For this review, use the dimensioned drawing (mm, ordinates from the lowest corner) and the shaded views. Coordinates: 2 decimals unless noted, no trailing zeros. Loops run counter-clockwise (first coordinate to the right, second up) from the corner with the lowest first, then second, coordinate; pieces in that order, holes last. Notation, with made-up numbers: (17.5, 15) -> (30.5, 15) arc R30 ccw to (30.5, 40) -> close; hole circle Ø1 at (53, 44.5). An arc over 180 degrees is marked (long way). Answer as a JSON object with one key per item and string values.
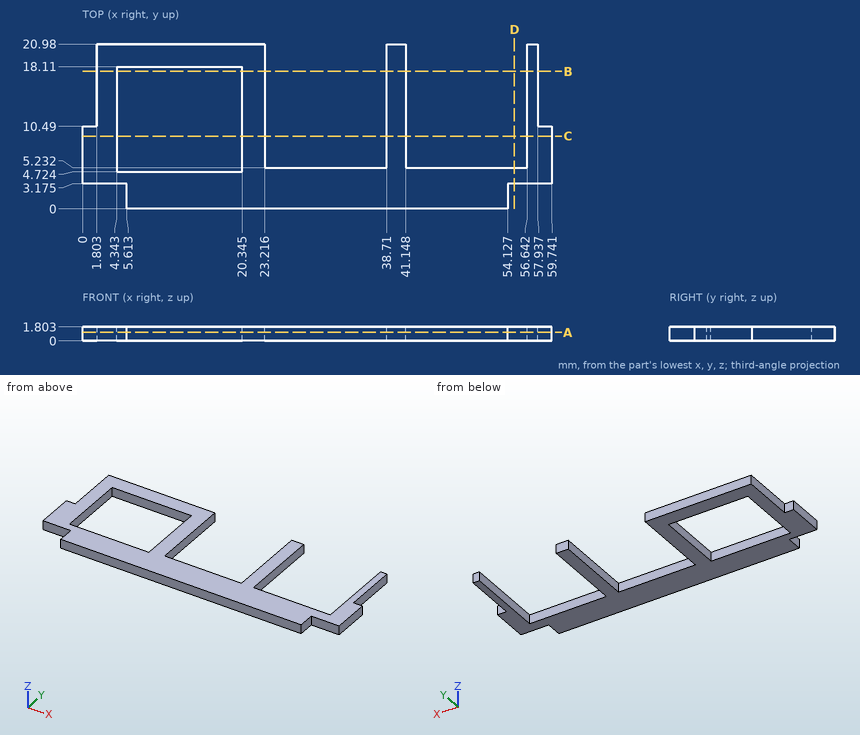
1) Wall thickness on probe 1 along X at (y, z) = (7.5, 1.15) (1 decimal); probe 2 along X at (y, z) = (12, 1.1) (1 decimal); probe 3 along X at (y, z) = (19.25, 0.7) (1 decimal): over which ranges is each line inside the solid? List them lowest first.
Completed:
{"probe 1": "0 to 4.3, 20.3 to 23.2, 38.7 to 41.1, 56.6 to 59.7", "probe 2": "1.8 to 4.3, 20.3 to 23.2, 38.7 to 41.1, 56.6 to 57.9", "probe 3": "1.8 to 23.2, 38.7 to 41.1, 56.6 to 57.9"}
2) Add section B-B, the plane y = 17.5. Give the boundary of the cut face in (x, z) (1 decimal).
Completed:
{"outline": "(1.8, 0) -> (4.3, 0) -> (4.3, 1.8) -> (1.8, 1.8) -> close; (20.3, 0) -> (23.2, 0) -> (23.2, 1.8) -> (20.3, 1.8) -> close; (38.7, 0) -> (41.1, 0) -> (41.1, 1.8) -> (38.7, 1.8) -> close; (56.6, 0) -> (57.9, 0) -> (57.9, 1.8) -> (56.6, 1.8) -> close"}
3) Add section C-C, the plane y = 9.25. Give the boundary of the cut face in (x, z) (1 decimal), and give its area (3 significant figures).
Completed:
{"outline": "(0, 0) -> (4.3, 0) -> (4.3, 1.8) -> (0, 1.8) -> close; (20.3, 0) -> (23.2, 0) -> (23.2, 1.8) -> (20.3, 1.8) -> close; (38.7, 0) -> (41.1, 0) -> (41.1, 1.8) -> (38.7, 1.8) -> close; (56.6, 0) -> (59.7, 0) -> (59.7, 1.8) -> (56.6, 1.8) -> close", "area": "23.0 mm²"}
4) Clearance check with flat-ended pins moving along their axes: pin 1 Ø0.9 at (y, z) = (18, 1) entering from +X; pin 2 Ø0.5 at (x, z) = (4, 1) entering from -Y (3 decimals); pin 3 Ø0.5 at (x, z) = (58.5, 0.5) entering from +Y. State where each tip first meets the part, or that it passes through.
Completed:
{"pin 1": "x = 57.94", "pin 2": "y = 3.175", "pin 3": "y = 10.49"}
5) Add section A-A, the plane z = 1.1. Give the boundary of the cut face in (x, y) (1 decimal).
Completed:
{"outline": "(0, 3.2) -> (5.6, 3.2) -> (5.6, 0) -> (54.1, 0) -> (54.1, 3.2) -> (59.7, 3.2) -> (59.7, 10.5) -> (57.9, 10.5) -> (57.9, 21) -> (56.6, 21) -> (56.6, 5.2) -> (41.1, 5.2) -> (41.1, 21) -> (38.7, 21) -> (38.7, 5.2) -> (23.2, 5.2) -> (23.2, 21) -> (1.8, 21) -> (1.8, 10.5) -> (0, 10.5) -> close; hole (4.3, 4.7) -> (20.3, 4.7) -> (20.3, 18.1) -> (4.3, 18.1) -> close"}
6) Add section D-D, the plane x = 55. Give the boundary of the cut face in (y, z) (1 decimal).
Completed:
{"outline": "(3.2, 0) -> (5.2, 0) -> (5.2, 1.8) -> (3.2, 1.8) -> close"}
